Autodesk Inventor part; units mm, degrees
ref_plane "YZ Plane" through (0, 0, 0) normal (1, 0, 0) x (0, 1, 0)
ref_plane "XZ Plane" through (0, 0, 0) normal (0, 1, 0) x (-1, 0, 0)
ref_plane "XY Plane" through (0, 0, 0) normal (0, 0, 1) x (1, 0, 0)
sketch "Szkic1" plane through (0, 0, 0) normal (0, 1, 0) x (-1, 0, 0)
  line L0 (55, -12.5) -> (-55, -12.5)
  line L1 (-55, -12.5) -> (-55, 20.5)
  line L2 (-43, 32.5) -> (43, 32.5)
  line L3 (55, 20.5) -> (55, -12.5)
  arc A0 (55, 20.5) -> (43, 32.5) centre (43, 20.5) ccw
  arc A1 (-43, 32.5) -> (-55, 20.5) centre (-43, 20.5) ccw
  point P0 (0, 0)
  point P1 (-55, 32.5)
  point P2 (55, 32.5)
  dimension "d0" = 110
  dimension "d1" = 45
  dimension "d2" = 12
extrude "Wyciągnięcie proste1" add sketch "Szkic1" along normal blind 12
sketch "Szkic2" plane through (0, 12, 0) normal (0, 1, 0) x (1, 0, 0)
  line L0 (55, 12.5) -> (-55, 12.5)
  line L1 (-55, 12.5) -> (55, 12.5)
  line L2 (55, 12.5) -> (55, 0.5)
  line L3 (55, 0.5) -> (-55, 0.5)
  line L4 (-55, 0.5) -> (-55, 12.5)
  point P0 (0, 0)
  dimension "d5" = 12
extrude "Wyciągnięcie proste2" add sketch "Szkic2" along normal blind 50
fillet "Zaokrąglenie1" radius 12 2 edges at (55, 62, -6.5) (-55, 62, -6.5)
sketch "Szkic3" plane through (-55, 12, -0.5) normal (0, 0, 1) x (1, 0, 0)
  line L0 (98, 50) -> (12, 50)
  line L1 (30, 50) -> (80, 50)
  line L2 (80, 50) -> (80, 40)
  line L3 (80, 40) -> (30, 40)
  line L4 (30, 40) -> (30, 50)
  line L5 (0, 0) -> (0, 38)
  line L6 (35, 40) -> (44, 0)
  line L7 (110, 0) -> (0, 0)
  line L8 (75, 40) -> (66, 0)
  line L9 (44, 0) -> (66, 0)
  line L10 (44, 0) -> (66, 0)
  line L11 (110, 0) -> (110, 38)
  point P0 (55, -12)
  point P1 (66, 0)
  dimension "d9" = 50
  dimension "d10" = 30
  dimension "d11" = 10
  dimension "d12" = 44
  dimension "d13" = 44
extrude "Wyciągnięcie proste3" add sketch "Szkic3" along normal blind 23
sketch "Szkic4" plane through (-55, 12, 22.5) normal (0, 0, 1) x (1, 0, 0)
  line L0 (98, 50) -> (12, 50)
  point P0 (55, -12)
  point P1 (55, 50)
hole "Otwór1" at (0, 62, 22.5) direction (0, 0, -1) diameter 30 end through all
sketch "Szkic5" plane through (-55, 12, -0.5) normal (0, 0, 1) x (1, 0, 0)
  arc A0 (12, 50) -> (0, 38) centre (12, 38) ccw
  arc A1 (110, 38) -> (98, 50) centre (98, 38) ccw
  point P0 (55, -12)
hole "Otwór2" at (-43, 50, -0.5) at (43, 50, -0.5) direction (0, 0, -1) diameter 12 end through all
sketch "Szkic6" plane through (0, 12, 0) normal (0, 1, 0) x (1, 0, 0)
  arc A0 (-55, -20.5) -> (-43, -32.5) centre (-43, -20.5) ccw
  arc A1 (43, -32.5) -> (55, -20.5) centre (43, -20.5) ccw
  point P0 (0, 0)
hole "Otwór3" at (-43, 12, 20.5) at (43, 12, 20.5) direction (0, -1, 0) diameter 12 end through all
sketch "Szkic7" plane through (0, 0, 0) normal (0, -1, 0) x (1, 0, 0)
  line L0 (-43, 32.5) -> (43, 32.5)
  line L1 (-30, 32.5) -> (30, 32.5)
  line L2 (30, 32.5) -> (30, 0)
  line L3 (30, 0) -> (-30, 0)
  line L4 (-30, 0) -> (-30, 32.5)
  point P0 (0, 0)
  dimension "d37" = 60
extrude "Wyciągnięcie proste4" cut sketch "Szkic7" against normal blind 6
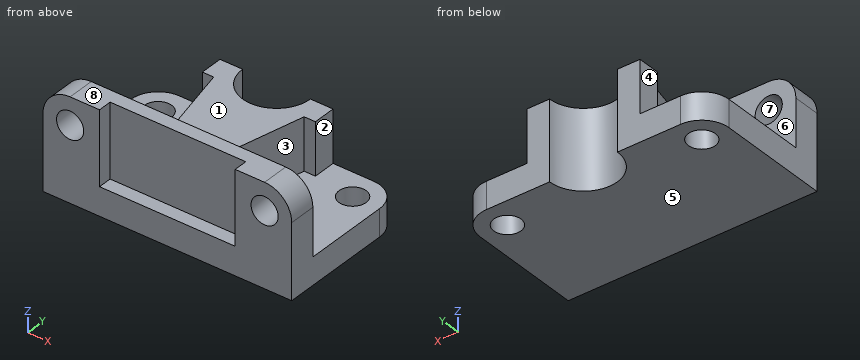
The listing builds one solid part. Answer for the finished solid, in the listing's coordinates (mm). Face numbers are marked on the shaded views. A direction names the side the tool comes from. Give positions to 0.01 mm unless a question says otherwise; leave off trailing zeros. Write each loop counter-clockwise with the first axis right and the second up, starting at its lowest first coordinate (ties: lowest second). Pieces come first, ordered by that corner, then holes. Notation, with made-up numbers: (11, 72.25) - (66, 72.25) arc R22 ccw to (66, 78.25) - close; hole circle Ø5 at (51, -2). An arc over 180 degrees is marked (long way). Use a Markdown table: item, result.
1. For a pull along Z with two mould halves and no side action, classify the marked faces 5, 6, 7 and 8 as released by +Z, released by -Z, zero draft, split by the parting line, or undercut.
Values follow:
| item | result |
|---|---|
| face 5 | released by -Z |
| face 6 | zero draft |
| face 7 | undercut |
| face 8 | released by +Z |
2. Section D-D on z = 3.5 is taken. Write down the section's boundary in (x, y).
Values follow:
| item | result |
|---|---|
| outline | (-55, 0) - (-30, 0) - (-30, 6) - (30, 6) - (30, 0) - (55, 0) - (55, 12) - (11, 12) - (20, 52) - (25, 52) - (25, 62) - (15, 62) arc R15 cw to (-15, 62) - (-25, 62) - (-25, 52) - (-20, 52) - (-11, 12) - (-55, 12) - close |
3. Section A-A on z = -9 is taken. Write down the section's boundary in (x, y), plus the area to 3 significant figures.
Values follow:
| item | result |
|---|---|
| outline | (-55, 0) - (55, 0) - (55, 50) arc R12 ccw to (43, 62) - (15, 62) arc R15 cw to (-15, 62) - (-43, 62) arc R12 ccw to (-55, 50) - close; hole circle Ø12 at (-43, 50); hole circle Ø12 at (43, 50) |
| area | 6,180 mm² |
4. A tool of negligible diameter and unlimited length cuts with its end or side. For the marked faces 1, 2, 3 and 4, from which of +Z, -Z, +X, -X, +Y, -Y can it reach the whole face along a straight path? Write none if from no direction.
Values follow:
| item | result |
|---|---|
| face 1 | +Z, +X, -X, +Y |
| face 2 | +Z, +X, +Y |
| face 3 | +Z, +X |
| face 4 | +Z, -X, +Y |
5. Each of these flat-tipped pins is pushed along its axis until it touches: P1, Ø16.5, axis at x = -3, z = 20.5, coming from the +Y side; P2, Ø9.5, axis at x = 43, y = 50, coming from the -Z side; P3, Ø8, axis at y = 59.5, z = 10.5, coming from the -X side; P4, Ø4, axis at y = 47, z = 18.5, coming from the +X side (3 decimals). Where does it stop, or does it pass through?
Values follow:
| item | result |
|---|---|
| P1 | stops at y = 52.08 |
| P2 | passes through |
| P3 | stops at x = -25 |
| P4 | stops at x = 19.325 |
6. Section C-C on y = 28 is taken. Write down the section's boundary in (x, z), plus the area to 3 significant figures.
Values follow:
| item | result |
|---|---|
| outline | (-55, -12.5) - (55, -12.5) - (55, -0.5) - (14.6, -0.5) - (14.6, 22.5) - (-14.6, 22.5) - (-14.6, -0.5) - (-55, -0.5) - close |
| area | 1,990 mm² |
7. Section B-B on x = 0 is taken. Write down the section's boundary in (y, z), plus the area to 3 significant figures.
Values follow:
| item | result |
|---|---|
| outline | (0, -12.5) - (47, -12.5) - (47, 22.5) - (12, 22.5) - (12, 32.5) - (6, 32.5) - (6, 0) - (0, 0) - close |
| area | 1,570 mm² |
8. Find the intervals of material crossed by probe 1 along X at (y, z) = (5.25, 20.5); probe 2 along X at (y, z) = (7, 20); probe 3 along X at (y, z) = (50, -6), in increasing order. Write a range as from..to.
Values follow:
| item | result |
|---|---|
| probe 1 | x = -55..-49, -37..-30, 30..37, 49..55 |
| probe 2 | x = -55..-48.98, -37.02..37.02, 48.98..55 |
| probe 3 | x = -55..-49, -37..-9, 9..37, 49..55 |
